Input: dimensioned drawing with shaded views. Units: mm. Origin: part minimum x, y, z. A direction names the side the tool comes from. Round coordinates to 2 decimals unless told otherwise and drop trailing zeros. Loops run counter-clockwise (first coordinate to the right, second up) from the corner with the lowest first, then second, coordinate; pieces in that order, holes last. Notation, with made-up numbers: M 60,-19.75 L 72,-19.75 A22 cw 72,-5.75 Z; hole C -36,64.5 d2. An arc over 180 degrees is marked long. Write each question's results on one line, items separated by ' | '. Start each with the question number.
1. Set-up query: the marked faces 1 and 2. Return all of +Z, -Z, +X, -X, +Y, -Y with unobstructed straight access to the full face (end or side cutting, diameter ignored); none if empty.
2. Section B-B on x = 18. Output: boundary loops of the cut face in (y, z), and give its area (3 significant figures).
3. Section C-C on z = 5.5. Output: boundary loops of the cut face in (x, y).
4. Section A-A on y = 17.5. Output: boundary loops of the cut face in (x, z), and give its area (3 significant figures).
5. Ray query, line 1 (X direction, y = 17.5, z = 8); line 2 (Z direction, x = 13, y = 7); line 3 (X direction, y = 10, z = 37.5). Return the intervals inside material, ascending.
6. Section D-D on y = 33. Output: boundary loops of the cut face in (x, z).
7. Contact query for flat-ended pins moving along their axis: pin 1 Ø5 at (x, y) = (19, 31) entering from -Z; pin 2 Ø5 at (y, z) = (23.5, 23) entering from +X. Output: stop coordinate, or through.
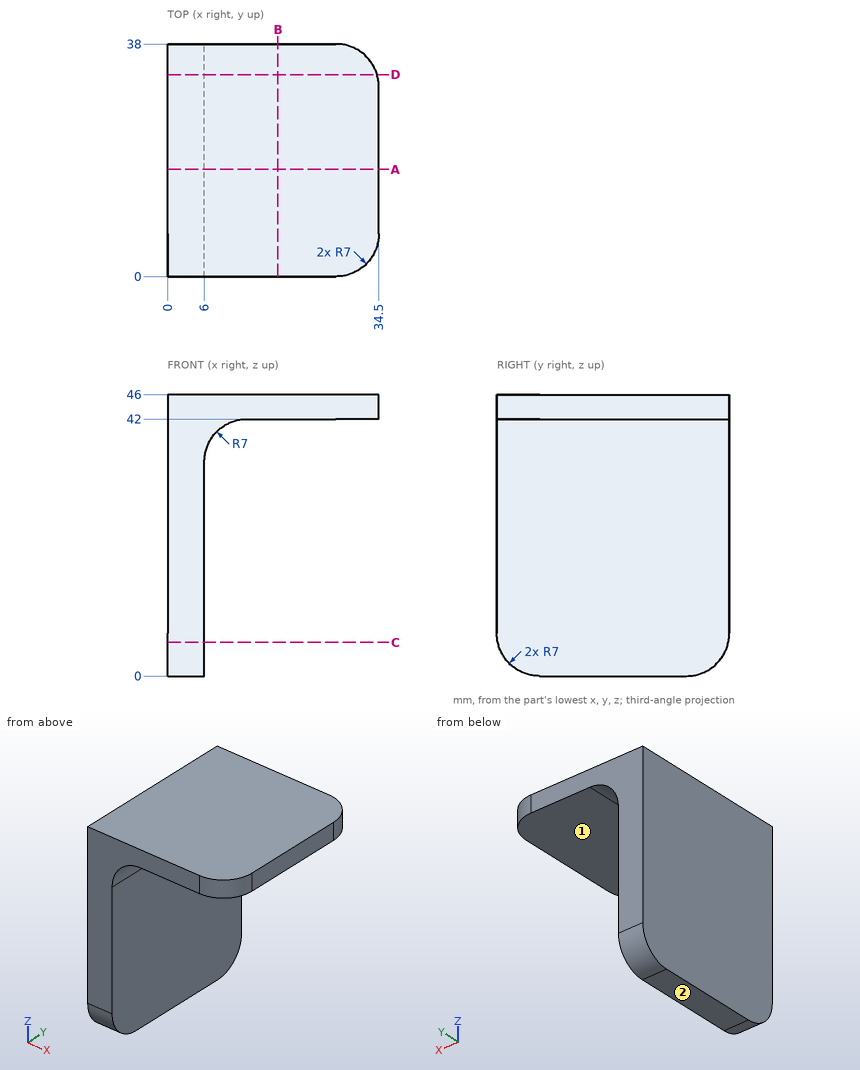
Taken from the geometry:
1) face 1: -Z, +X, +Y, -Y | face 2: -Z, +X, -X, +Y, -Y
2) outline: M 0,42 L 38,42 L 38,46 L 0,46 Z | area: 152 mm^2
3) outline: M 0,0.16 L 6,0.16 L 6,37.84 L 0,37.84 Z
4) outline: M 0,0 L 6,0 L 6,35 A7 cw 13,42 L 34.5,42 L 34.5,46 L 0,46 Z | area: 401 mm^2
5) line 1: 0 to 6 | line 2: 42 to 46 | line 3: 0 to 6.46
6) outline: M 0,0.29 L 6,0.29 L 6,35 A7 cw 13,42 L 34.21,42 L 34.21,46 L 0,46 Z
7) pin 1: z = 42 | pin 2: x = 6
